Model file for the job. Use its own axes, mm. A direction names the side the tool comes from. Give positions to 0.01 mm unless a question says otherwise; leave off trailing zeros. Loops run counter-clockwise (first coordinate to the right, second up) from the corner with the lowest first, then second, coordinate; pieces in that order, holes last. Notation, with made-up numbers: (-19, -7.5) - (19, -7.5) arc R32 ccw to (19, 29.5) - close; hole circle Ø6 at (66, -5). An arc over 180 degrees is marked (long way). Answer as CSV lines item,"result". Start each with the question number.
Item 1: Pin check, flat tip, straight feed: pin 1 (2.5 mm diameter, centred on x = 8.5, y = 11, fed in from -Z). Stop position of the tip, or through.
Item 2: Drill centre lines: L1, parallel to X at y = 12.5, z = 0.65; L2, parallel to X at y = 12.5, z = 2.45; L3, parallel to Y at x = 6.35, z = 3.85. Where is each one in solid material? Low to high. Write a range as from..to.
Item 3: Saw through at D-D on x = 6.35. Give the cut face in (y, z), plus the area to 3 significant figures.
Item 4: Saw through at B-B on x = 94.85. Give the cut face in (y, z).
Item 5: Saw through at C-C on y = 12.5. State how many separate pieces and enclosed holes the cut face has, plus the area to 3 significant figures.
Item 6: Saw through at A-A on z = 2.9. Give the cut face in (x, y), plus the area to 3 significant figures.
Item 7: Tool access for faces 4 (the flat face through (95, 15, 1)), 5 (the cylindrical face through (93.33, 10.84, 3.03)): list every direction of +Z, -Z, +X, -X, +Y, -Y with a clear straight run to the whole face (end or side of a thin tool).
Item 8: Pull direction X, two halves, no side cores. Call faces 1 (the flat face through (0, 13, 2)), 2 (the cylindrical face through (137.79, 11.51, 0.51)), 3 (the flat face through (71, 25, 2)): pulls with the +X half, pulls with the -X half, needs draft (parallel to the pull), parting line crosses it, or undercut.
Autodesk Fusion 360 part; units mm, degrees
sketch "Sketch1" plane through (0, 0, 0) normal (0, 0, 1) x (1, 0, 0)
  line L0 (0, 0) -> (139.7, 0)
  line L1 (139.7, 0) -> (139.7, 25)
  line L2 (139.7, 25) -> (0, 25)
  line L3 (0, 25) -> (0, 0)
  dimension "d1" = 139.7
  dimension "d2" = 25
extrude "Extrude1" add sketch "Sketch1" along normal blind 5
sketch "Sketch2" plane through (0, 0, 0) normal (0, 0, 1) x (1, 0, 0)
  point P0 (6.35, 12.5)
  point P1 (133.35, 12.5)
hole "Hole1" at (6.35, 12.5, 0) at (133.35, 12.5, 0) direction (0, 0, 1) diameter 5.5 depth 13 tip angle 118 counterbore diameter 9.1 counterbore depth 1
sketch "Sketch3" plane through (0, 0, 0) normal (0, 0, -1) x (1, 0, 0)
  circle A0 centre (6.35, -12.5) radius 4.55
  circle A1 centre (133.35, -12.5) radius 4.55
  line L0 (0, 0) -> (0, -25)
  line L1 (0, -25) -> (139.7, -25)
  line L2 (139.7, -25) -> (139.7, 0)
  line L3 (139.7, 0) -> (0, 0)
  point P0 (94.85, -12.5)
  point P1 (44.85, -12.5)
hole "Hole2" at (94.85, 12.5, 0) at (44.85, 12.5, 0) direction (0, 0, 1) diameter 4.5 end through all counterbore diameter 7.5 counterbore depth 1
Responses:
1,pin 1,"z = 1"
2,L1,"0..1.8, 10.9..41.1, 48.6..91.1, 98.6..128.8, 137.9..139.7"
2,L2,"0..3.6, 9.1..42.6, 47.1..92.6, 97.1..130.6, 136.1..139.7"
2,L3,"0..9.75, 15.25..25"
3,outline,"(0, 0) - (7.95, 0) - (7.95, 1) - (9.75, 1) - (9.75, 5) - (0, 5) - close; (15.25, 1) - (17.05, 1) - (17.05, 0) - (25, 0) - (25, 5) - (15.25, 5) - close"
3,area,"93.9 mm2"
4,outline,"(0, 0) - (8.75, 0) - (8.75, 1) - (10.25, 1) - (10.25, 5) - (0, 5) - close; (14.75, 1) - (16.25, 1) - (16.25, 0) - (25, 0) - (25, 5) - (14.75, 5) - close"
5,separate pieces,"5"
5,enclosed holes,"0"
5,area,"585 mm2"
6,outline,"(0, 0) - (139.7, 0) - (139.7, 25) - (0, 25) - close; hole circle Ø5.5 at (6.35, 12.5); hole circle Ø4.5 at (44.85, 12.5); hole circle Ø4.5 at (94.85, 12.5); hole circle Ø5.5 at (133.35, 12.5)"
6,area,"3,410 mm2"
7,face 4,"-Z"
7,face 5,"+Z, -Z"
8,face 1,"pulls with the -X half"
8,face 2,"undercut"
8,face 3,"needs draft"
